For this review, take the finished solid that the model builds, in its own axes (mm). A direction names the side the tool comes from. Coordinates: 2 decimals unless noted, no trailing zeros. Loops run counter-clockwise (first coordinate to the right, second up) from the corner with the lowest first, then second, coordinate; pieces in that order, holes last. Notation, with made-up numbers: (36, 44) -> (66, 44) arc R12 cw to (66, 66) -> close; hole circle Ø9 at (41, 77.5). An arc over 180 degrees is marked (long way). One line per item, written item: value.
from build123d import *

# Parameters (mm, degrees)
F3_R     = 23.5045362994
F4_DEPTH = 76.2


with BuildPart() as f1:
    # F0 (on Top) → F1 (revolve)
    with BuildSketch(Plane.XY):
        Polygon((573.0409642621, -553.5393390198), (585.7409642621, -553.5393390198), (585.7409642621, -518.0866146582), (542.4275865968, -518.0866146582), (512.1499083626, -496.5325579214), (512.1499083626, -311.0723252855), (469.6844318455, -269.9765585894), (469.6844318455, -197.0943934766), (519.4383481781, -154.4892936945), (519.4383481781, -107.0225714794), (586.8421554444, -77.3644662998), (586.8421554444, 0), (574.1421554444, 0), (574.1421554444, -61.8945817717), (506.7383481781, -90.8532650404), (506.7383481781, -146.9035498934), (456.9844318455, -188.7616498797), (456.9844318455, -275.1079445892), (499.4499083626, -315.4920612499), (499.4499083626, -503.081022234), (538.3688470547, -530.7866146582), (573.0409642621, -530.7866146582), align=None)
    revolve(axis=Axis((0, -57.5910839191, 0), (0, -1, 0)))

    # F3 (on offset) → F4 (join)
    with BuildSketch(Plane.XZ.offset(190.5)):
        with BuildLine():
            Line((-381.5941034135, -251.4372907688), (-54.9773815999, -114.4835687443))
            ThreePointArc((-54.9773815999, -114.4835687443), (-109.9852262806, -63.5), (-126.6343696484, 9.6299752731))
            Line((-126.6343696484, 9.6299752731), (-408.5481329713, -204.7515421061))
            ThreePointArc((-408.5481329713, -204.7515421061), (-395.7601271122, -228.4922159227), (-381.5941034135, -251.4372907688))
        make_face()
        with BuildLine():
            ThreePointArc((-71.6569880485, 104.8535934712), (-37.5006241892, 121.3371467664), (0, 127))
            Line((0, 127), (0, 456.9844318455))
            ThreePointArc((0, 456.9844318455), (-13.4828844014, 456.785488799), (-26.9540295578, 456.1888328749))
            Line((-26.9540295578, 456.1888328749), (-71.6569880485, 104.8535934712))
        make_face()
        with BuildLine():
            ThreePointArc((0, 127), (37.5006241892, 121.3371467664), (71.6569880485, 104.8535934712))
            Line((71.6569880485, 104.8535934712), (26.9540295578, 456.1888328749))
            ThreePointArc((26.9540295578, 456.1888328749), (13.4828844014, 456.785488799), (0, 456.9844318455))
            Line((0, 456.9844318455), (0, 127))
        make_face()
        with BuildLine():
            ThreePointArc((126.6343696484, 9.6299752731), (126.9085594933, 4.8184569448), (127, 0))
            ThreePointArc((127, 0), (107.4968080065, -67.6271858679), (54.9773815999, -114.4835687443))
            Line((54.9773815999, -114.4835687443), (381.5941034135, -251.4372907688))
            ThreePointArc((381.5941034135, -251.4372907688), (395.7601271122, -228.4922159227), (408.5481329713, -204.7515421061))
            Line((408.5481329713, -204.7515421061), (126.6343696484, 9.6299752731))
        make_face()
        with BuildLine():
            ThreePointArc((54.9773815999, -114.4835687443), (107.4968080065, -67.6271858679), (127, 0))
            ThreePointArc((127, 0), (126.9085594933, 4.8184569448), (126.6343696484, 9.6299752731))
            ThreePointArc((126.6343696484, 9.6299752731), (109.9852262806, 63.5), (71.6569880485, 104.8535934712))
            ThreePointArc((71.6569880485, 104.8535934712), (37.5006241892, 121.3371467664), (0, 127))
            ThreePointArc((0, 127), (-37.5006241892, 121.3371467664), (-71.6569880485, 104.8535934712))
            ThreePointArc((-71.6569880485, 104.8535934712), (-109.9852262806, 63.5), (-126.6343696484, 9.6299752731))
            ThreePointArc((-126.6343696484, 9.6299752731), (-109.9852262806, -63.5), (-54.9773815999, -114.4835687443))
            ThreePointArc((-54.9773815999, -114.4835687443), (0, -127), (54.9773815999, -114.4835687443))
        make_face()
        with Locations((-45.8940714598, -52.665323019)):
            Circle(F3_R, mode=Mode.SUBTRACT)
        with Locations((52.665323019, -45.8940714598)):
            Circle(F3_R, mode=Mode.SUBTRACT)
        with Locations((-52.665323019, 45.8940714598)):
            Circle(F3_R, mode=Mode.SUBTRACT)
        with Locations((45.8940714598, 52.665323019)):
            Circle(F3_R, mode=Mode.SUBTRACT)
    extrude(amount=F4_DEPTH)


solid = f1.part
1. For faces 3 (the cylindrical face through (-113, -130, -507)), 4 (the flat face through (512, -530.787, -167)), 5 (the cylindrical face through (-109.85, -119.27, -494.69)), 6 (the flat face through (-220.57, -228.07, -183.92)), list the 3-axis set-ups (+Z, -Z, +X, -X, +Y, -Y) from which the entire face can be reached by the end or side of a thin tool; tool diameter is ignored.
Return value:
face 3: none
face 4: -Y
face 5: +Y
face 6: +Y, -Y
2. The part is to be moulded in two halves that separate along Z. For faces 1 (the conical face through (449.96, -271.97, 141.7)), 2 (the conical face through (-99.641, -277.634, -448.711)), say which applies: pulls with the +Z half, pulls with the -Z half, needs draft (parallel to the pull), parting line crosses it, or undercut.
Return value:
face 1: parting line crosses it
face 2: undercut
3. Take a section at B-B, the plane x = -234.5. Give the number of separate pieces and of enclosed holes in the cut face, and give its area (3 significant figures).
Return value:
separate pieces: 3
enclosed holes: 0
area: 30,100 mm2
4. Insertion check: pin 1 Ø10 at (x, z) = (352, -154) entering from -Y; pin 2 Ø10 at (y, z) = (-449.5, -343.5) entering from -X; pin 3 Ø8 at (x, z) = (-278.5, 382) entering from +Y; pin 4 Ø4 at (x, y) = (27.5, -423.5) entering from -Z. Each pin has a flat end and moves straight along its axis. Give the tip position at first contact, or say it passes through.
Return value:
pin 1: passes through
pin 2: stops at x = -384.34
pin 3: stops at y = -172.14
pin 4: stops at z = -511.51
5. Take a section at A-A, the plane y = -402. Give the boundary of the cut face in (x, z), and give its area (3 significant figures).
Return value:
outline: circle Ø1024.3 at (0, 0); hole circle Ø998.9 at (0, 0)
area: 40,400 mm2
6. Take a section at D-D, the plane y = -41. Give the boundary of the cut face in (x, z), and give its area (3 significant figures).
Return value:
outline: circle Ø1173.68 at (0, 0); hole circle Ø1148.28 at (0, 0)
area: 46,300 mm2
7. To check wall thickness, follow probe 1 along Z at (x, y) = (0, -18); probe 2 along Y at (x, z) = (-238, -135); probe 3 along Z at (x, y) = (142.5, -236.5). State the ranges of each line that lie inside material, in increasing order. Write a range as from..to.
Return value:
probe 1: z = -586.84..-574.14, 574.14..586.84
probe 2: y = -266.7..-190.5
probe 3: z = -447.55..-434.2, -151.18..-2.44, 434.2..447.55
